Could you check a few things on this model? Use its own coordinates, in mm. A direction names the side the tool comes from. Round coordinates to 2 decimals unless told otherwise and drop trailing zeros. Write each loop counter-clockwise with the first axis right and the second up, starting at its lowest first coordinate (ties: lowest second). Pieces come first, ordered by that corner, then holes. Notation, with made-up numbers: (-4, 38.5) -> (9, 38.5) arc R15 ccw to (9, 65.5) -> close; hole circle Ø8 at (19, 87). An arc over 180 degrees is marked (long way). Return JSON: item names as keys, results as strings.
from build123d import *

# Parameters (mm, degrees)
SKETCH3_W           = 114.3
SKETCH3_H           = 127
BOSS_EXTRUDE1_DEPTH = 8.89
SKETCH5_R           = 1.524
CUT_EXTRUDE1_DEPTH  = 172.092145056
SHELL2_T            = -6.35
SKETCH6_W           = 88.9
SKETCH6_H           = 127
BOSS_EXTRUDE2_DEPTH = 88.9
SKETCH8_R           = 7.874
CUT_EXTRUDE2_DEPTH  = 190.774719338
CUT_EXTRUDE3_DEPTH  = 197.866386415
FILLET1_R           = 5.08
CUT_EXTRUDE4_DEPTH  = 165.086159295
CUT_EXTRUDE5_DEPTH  = 190.725297655
FILLET2_R           = 1.27
SKETCH20_W          = 127
SKETCH20_H          = 20.338660629
CUT_EXTRUDE7_DEPTH  = 2.54
DRAFT6_DEPTH        = 114.3
DRAFT6_START        = -128
DRAFT6_2_DEPTH      = 129
DRAFT7_ANGLE        = 3


with BuildPart() as part:
    # Sketch3 → Boss-Extrude1 (new body)
    with BuildSketch(Plane(origin=(0, 0, 0), x_dir=(0, 1, 0), z_dir=(0, 0, 1))):
        with Locations((57.15, 63.5)):
            Rectangle(SKETCH3_W, SKETCH3_H)
    extrude(amount=BOSS_EXTRUDE1_DEPTH)

    # Sketch5 → Cut-Extrude1 (cut, through all)
    with BuildSketch(Plane.XY.offset(8.89)):
        with Locations((-119.38, 7.62)):
            Circle(SKETCH5_R)
        with Locations((-7.62, 7.62)):
            Circle(SKETCH5_R)
        with Locations((-119.38, 106.68)):
            Circle(SKETCH5_R)
        with Locations((-7.62, 106.68)):
            Circle(SKETCH5_R)
    extrude(amount=-CUT_EXTRUDE1_DEPTH, mode=Mode.SUBTRACT)

    # Shell2
    shell2_openings = [part.faces().sort_by_distance(p)[0] for p in [
        (-63.5, 57.15, 0),
    ]]
    offset(amount=SHELL2_T, openings=shell2_openings)

    # Sketch6 → Boss-Extrude2 (add)
    with BuildSketch(Plane(origin=(0, 0, 8.89), x_dir=(0, -1, 0), z_dir=(0, 0, 1))):
        with Locations((-57.15, -63.5)):
            Rectangle(SKETCH6_W, SKETCH6_H)
    extrude(amount=BOSS_EXTRUDE2_DEPTH)

    # Sketch8 → Cut-Extrude2 (cut, through all)
    with BuildSketch(Plane(origin=(0, 101.6, 0), x_dir=(-1, 0, 0), z_dir=(0, 1, 0))):
        with Locations(Location((63.5, 85.09, 0), (0, 0, 90))):
            Circle(SKETCH8_R)
        Polygon((55.88, 97.79), (0, 97.79), (0, 72.39), align=None)
        Polygon((71.12, 97.79), (127, 97.79), (127, 72.39), align=None)
    extrude(amount=-CUT_EXTRUDE2_DEPTH, mode=Mode.SUBTRACT)

    # Sketch9 → Cut-Extrude3 (cut, through all)
    with BuildSketch(Plane(origin=(-127, 0, 0), x_dir=(0, -1, 0), z_dir=(-1, 0, 0))):
        Polygon((-67.31, 97.79), (-46.99, 97.79), (-46.99, 59.69), (-27.718040346, 8.974316699), (-86.47043568, 9.267800843), (-67.31, 59.69), align=None)
        Polygon((-77.47, 97.79), (-77.47, 72.39), (-101.6, 8.89), (-101.6, 97.79), align=None)
        Polygon((-36.83, 97.79), (-36.83, 72.39), (-12.7, 8.89), (-12.7, 97.79), align=None)
    extrude(amount=-CUT_EXTRUDE3_DEPTH, mode=Mode.SUBTRACT)

    # Fillet1
    fillet1_edges = [part.edges().sort_by_distance(p)[0] for p in [
        (-63.5, 27.718040346, 8.974316699),
        (-63.5, 86.47043568, 9.267800843),
    ]]
    fillet(fillet1_edges, radius=FILLET1_R)

    # Sketch16 → Cut-Extrude4 (cut, through all)
    with BuildSketch(Plane(origin=(0, 78.63701503, 29.882065711), x_dir=(1, 0, 0), z_dir=(0, -0.9347835805883491, -0.3552177606235725))):
        Polygon((-12.7, -14.726847163), (-114.3, -14.726847163), (-63.5, 26.915400792), align=None)
        Polygon((-12.7, 26.915400792), (-50.8, 26.915400792), (-12.7, -4.316285174), align=None)
        Polygon((-114.3, -4.316285174), (-114.3, 26.915400792), (-76.2, 26.915400792), align=None)
    extrude(amount=-CUT_EXTRUDE4_DEPTH, mode=Mode.SUBTRACT)

    # Sketch17 → Cut-Extrude5 (cut, through all)
    with BuildSketch(Plane(origin=(0, 21.240650122, -8.071447046), x_dir=(-1, 0, 0), z_dir=(0, 0.934783580588349, -0.3552177606235728))):
        Polygon((114.3, 25.842533623), (12.7, 25.842533623), (63.5, 67.484781577), align=None)
        Polygon((114.3, 67.484781577), (76.2, 67.484781577), (114.3, 36.253095611), align=None)
        Polygon((12.7, 36.253095611), (12.7, 67.484781577), (50.8, 67.484781577), align=None)
    extrude(amount=-CUT_EXTRUDE5_DEPTH, mode=Mode.SUBTRACT)

    # Fillet2
    fillet2_edges = [part.edges().sort_by_distance(p)[0] for p in [
        (-76.2, 75.623722461, 57.530204051),
        (-114.3, 86.71777201, 28.335336816),
        (-114.3, 75.623722461, 57.530204051),
        (-12.7, 75.623722461, 57.530204051),
        (-12.7, 86.71777201, 28.335336816),
        (-50.8, 75.623722461, 57.530204051),
        (-12.7, 90.415788526, 18.603714404),
        (-63.5, 75.623722461, 57.530204051),
        (-114.3, 90.415788526, 18.603714404),
        (-50.8, 38.664907284, 57.500282325),
        (-12.7, 27.570857734, 28.30541509),
        (-12.7, 38.664907284, 57.500282325),
        (-114.3, 38.664907284, 57.500282325),
        (-114.3, 27.570857734, 28.30541509),
        (-76.2, 38.664907284, 57.500282325),
        (-63.5, 38.664907284, 57.500282325),
        (-114.3, 23.872841218, 18.573792679),
        (-12.7, 23.872841218, 18.573792679),
        (-120.65, 57.15, 2.54),
    ]]
    fillet(fillet2_edges, radius=FILLET2_R)

    # Sketch20 → Cut-Extrude7 (cut)
    with BuildSketch(Plane(origin=(0, -0.044136403, 8.8356371), x_dir=(1, 0, 0), z_dir=(0, -0.004995208795198877, 0.9999875238667193))):
        with Locations((-63.5, 57.456908074)):
            Rectangle(SKETCH20_W, SKETCH20_H)
    extrude(amount=-CUT_EXTRUDE7_DEPTH, mode=Mode.SUBTRACT)

    # Draft6: read off the stored shape, not the designer's step
    # Draft6 outline → Draft6 (cut)
    with BuildSketch(Plane(origin=(0, 0, 0), x_dir=(1, 0, 0), z_dir=(0, 1, 0))):
        Polygon((-120.404404826, -75.387997806), (-127, 0), (-127, -72.39), align=None)
        Polygon((0, 0), (-6.595595174, -75.387997806), (0, -72.39), align=None)
    extrude(amount=DRAFT6_DEPTH, mode=Mode.SUBTRACT)

    # Draft6 2 outline → Draft6 2 (cut)
    with BuildSketch(Plane.YZ.offset(DRAFT6_START)):
        Polygon((0, 0), (0.777774219, 8.89), (0, 8.89), align=None)
        Polygon((113.522225781, 8.89), (114.3, 0), (114.3, 8.89), align=None)
    extrude(amount=DRAFT6_2_DEPTH, mode=Mode.SUBTRACT)

    # Draft7
    draft7_faces = [part.faces().sort_by_distance(p)[0] for p in [
        (-63.5, 46.99, 74.057550682),
        (-63.5, 67.31, 74.057550682),
    ]]
    draft(draft7_faces, Plane(origin=(0, 0, 59.69), x_dir=(0, 1, 0), z_dir=(0, 0, 1)), DRAFT7_ANGLE)


solid = part.part
1) I want a section at A-A, the plane z = 85.09. Please give me the cut outline in (x, y).
Return value:
{"outline": "(-99.06, 36.83) -> (-71.37, 36.83) -> (-71.37, 45.66) -> (-99.06, 45.66) -> close; (-99.06, 68.64) -> (-71.37, 68.64) -> (-71.37, 77.47) -> (-99.06, 77.47) -> close; (-55.63, 36.83) -> (-27.94, 36.83) -> (-27.94, 45.66) -> (-55.63, 45.66) -> close; (-55.63, 68.64) -> (-27.94, 68.64) -> (-27.94, 77.47) -> (-55.63, 77.47) -> close"}
2) Will these pins go through, and if not, where does the flat tip stop? pin 1 Ø8 at (y, z) = (36.5, 20.5) entering from -X; pin 2 Ø25 at (y, z) = (38.5, 38) entering from +X; pin 3 Ø4 at (x, y) = (-109, 77) entering from -Z; pin 4 Ø1.3 at (x, z) = (-52, 2) entering from +Y.
Return value:
{"pin 1": "through", "pin 2": "x = -2.3", "pin 3": "z = 2.54", "pin 4": "y = 114.18"}
3) I want a section at C-C, the plane z = 50.5. Count the separate pieces of the cut face and the enclosed holes in it, and give its area (3 significant figures).
Return value:
{"separate pieces": "8", "enclosed holes": "0", "area": "1,260 mm²"}
4) Thinking about a two-plate mould opening in X: for faces 1 (the face through (-113.918, 75.844, 57.227)), 2 (the face through (-78.167, 72.025, 47.281)), 3 (the face through (-2.794, 35.717, 31.934)), which applies, pulls with the +X half, pulls with the -X half, needs draft (parallel to the pull), parting line crosses it, or undercut?
Return value:
{"face 1": "undercut", "face 2": "needs draft", "face 3": "pulls with the +X half"}
5) If I drill on probe 1 along Y at (x, z) = (-53, 76); probe 2 along Y at (x, z) = (-119.38, 4.75); probe 3 along Y at (x, z) = (-119.38, 5.75), over which ranges is the centre line in solid material (lowest first)? Write a range as [from, to].
Return value:
{"probe 1": "[36.83, 46.14], [68.16, 77.47]", "probe 2": "[0.42, 6.1], [9.14, 105.16], [108.2, 113.88]", "probe 3": "[0.5, 6.1], [9.14, 105.16], [108.2, 113.8]"}
6) I want a section at B-B, the plane y = 60. Please give me the cut outline in (x, z).
Return value:
{"outline": "(-127, 0) -> (-120.65, 0) -> (-120.65, 1.27) arc R1.27 cw to (-119.38, 2.54) -> (-6.35, 2.54) -> (-6.35, 0) -> (0, 0) -> (-0.58, 6.6) -> (-126.42, 6.6) -> close"}
7) For faces 4 (the face through (-13.082, 75.844, 57.227)), 5 (the face through (-62.839, 90.324, 18.569)), 6 (the face through (-6.21, 7.04, 4.51)), 7 (the face through (-123.687, 35.717, 37.87)), 8 (the face through (-62.62, 30.96, 11.14)), which set-ups out of +Z, -Z, +X, -X, +Y, -Y let a thin tool reach every point of the face, with its end or its side?
Return value:
{"face 4": "+Y", "face 5": "none", "face 6": "+Z, -Z", "face 7": "+Z, -X, +Y, -Y", "face 8": "+X, -X"}
